from build123d import *

# Parameters (mm, degrees)
SKETCH1_R           = 1.5
SKETCH1_R_2         = 2.5
BOSS_EXTRUDE1_DEPTH = 3
CUT_EXTRUDE1_DEPTH  = 3
FILLET1_R           = 3
CHAMFER4_SIZE       = 15
CHAMFER5_DEPTH      = 3
SKETCH8_R           = 2
CUT_EXTRUDE4_DEPTH  = 10
SKETCH10_W          = 65
SKETCH10_H          = 15
BOSS_EXTRUDE2_DEPTH = 3
SKETCH9_W           = 6
SKETCH9_H           = 5
CUT_EXTRUDE5_DEPTH  = 10
FILLET2_R           = 3
SKETCH11_W          = 40
SKETCH11_H          = 3
CUT_EXTRUDE6_DEPTH  = 10


with BuildPart() as part:
    # Sketch1 → Boss-Extrude1 (new body)
    with BuildSketch(Plane.XY):
        with BuildLine():
            Line((40.5, -40), (44.5, -40))
            Line((44.5, -40), (47.5, -37))
            Line((47.5, -37), (47.5, 10))
            Line((47.5, 10), (47.5, 15))
            Line((47.5, 15), (52.5, 15))
            Line((52.5, 15), (70, 15))
            ThreePointArc((70, 15), (73.535533906, 16.464466094), (75, 20))
            Line((75, 20), (75, 60))
            ThreePointArc((75, 60), (73.535533906, 63.535533906), (70, 65))
            Line((70, 65), (-70, 65))
            ThreePointArc((-70, 65), (-73.535533906, 63.535533906), (-75, 60))
            Line((-75, 60), (-75, 20))
            ThreePointArc((-75, 20), (-73.535533906, 16.464466094), (-70, 15))
            Line((-70, 15), (-52.5, 15))
            Line((-52.5, 15), (-47.5, 15))
            Line((-47.5, 15), (-47.5, 10))
            Line((-47.5, 10), (-47.5, -37))
            Line((-47.5, -37), (-44.5, -40))
            Line((-44.5, -40), (-40.5, -40))
            Line((-40.5, -40), (-37.5, -37))
            Line((-37.5, -37), (-37.5, 10))
            ThreePointArc((-37.5, 10), (-36.035533906, 13.535533906), (-32.5, 15))
            Line((-32.5, 15), (32.5, 15))
            ThreePointArc((32.5, 15), (36.035533906, 13.535533906), (37.5, 10))
            Line((37.5, 10), (37.5, -37))
            Line((37.5, -37), (40.5, -40))
        make_face()
        with Locations((-42.5, -20)):
            Circle(SKETCH1_R, mode=Mode.SUBTRACT)
        with Locations((-42.5, -35)):
            Circle(SKETCH1_R, mode=Mode.SUBTRACT)
        with Locations((42.5, -20)):
            Circle(SKETCH1_R, mode=Mode.SUBTRACT)
        with Locations((42.5, -35)):
            Circle(SKETCH1_R, mode=Mode.SUBTRACT)
        with Locations((60, 40)):
            Circle(SKETCH1_R_2, mode=Mode.SUBTRACT)
        with Locations((15, 60)):
            Circle(SKETCH1_R, mode=Mode.SUBTRACT)
        with Locations(Location((-15, 60, 0), (0, 0, 180))):
            Circle(SKETCH1_R, mode=Mode.SUBTRACT)
        with Locations(Location((-60, 40, 0), (0, 0, 180))):
            Circle(SKETCH1_R_2, mode=Mode.SUBTRACT)
    extrude(amount=BOSS_EXTRUDE1_DEPTH)

    # Sketch3 → Cut-Extrude1 (cut)
    with BuildSketch(Plane.XY.offset(3)):
        Polygon((65, 50), (65, 30), (47.5, 30), (47.5, 15), (75, 15), (75, 23.034767996), (75, 32.364095159), (75, 65), (47.5, 65), (47.5, 50), align=None)
        Polygon((-47.5, 65), (-75, 65), (-75, 32.364095159), (-75, 23.034767996), (-75, 15), (-47.5, 15), (-47.5, 30), (-65, 30), (-65, 50), (-47.5, 50), align=None)
    extrude(amount=-CUT_EXTRUDE1_DEPTH, mode=Mode.SUBTRACT)

    # Fillet1
    fillet1_edges = [part.edges().sort_by_distance(p)[0] for p in [
        (65, 50, 1.5),
        (65, 30, 1.5),
        (-65, 50, 1.5),
        (-65, 30, 1.5),
    ]]
    fillet(fillet1_edges, radius=FILLET1_R)

    # Chamfer4
    chamfer4_edges = [part.edges().sort_by_distance(p)[0] for p in [
        (47.5, 65, 1.5),
        (-47.5, 65, 1.5),
    ]]
    chamfer(chamfer4_edges, length=CHAMFER4_SIZE - 0.0001)  # a hair under: the kernel refuses the full size

    # Chamfer5: read off the stored shape, not the designer's step
    # Chamfer5 outline → Chamfer5 (add)
    with BuildSketch(Plane.XY):
        with BuildLine():
            Line((47.5, 15.006945785), (62.083333333, 30.001157631))
            ThreePointArc((62.083333333, 30.001157631), (62.041670687, 30.000289422), (62, 30))
            Line((62, 30), (47.5, 30))
            Line((47.5, 30), (47.5, 15.006945785))
        make_face()
        with BuildLine():
            Line((-62.083333333, 30.001157631), (-47.5, 15.006945785))
            Line((-47.5, 15.006945785), (-47.5, 30))
            Line((-47.5, 30), (-62, 30))
            ThreePointArc((-62, 30), (-62.041670687, 30.000289422), (-62.083333333, 30.001157631))
        make_face()
    extrude(amount=CHAMFER5_DEPTH)

    # Sketch8 → Cut-Extrude4 (cut)
    with BuildSketch(Plane.XY.offset(3)):
        with Locations((-17.5, 43.444515249)):
            Circle(SKETCH8_R)
        with Locations((17.5, 43.444515249)):
            Circle(SKETCH8_R)
    extrude(amount=-CUT_EXTRUDE4_DEPTH, mode=Mode.SUBTRACT)

    # Sketch10 → Boss-Extrude2 (add)
    with BuildSketch(Plane.XY.offset(3)):
        with Locations((0, 72.5)):
            Rectangle(SKETCH10_W, SKETCH10_H)
    extrude(amount=-BOSS_EXTRUDE2_DEPTH)

    # Sketch9 → Cut-Extrude5 (cut)
    with BuildSketch(Plane.XY.offset(3)):
        with Locations((-25.5, 74.5)):
            Rectangle(SKETCH9_W, SKETCH9_H)
        with Locations((25.5, 74.5)):
            Rectangle(SKETCH9_W, SKETCH9_H)
    extrude(amount=-CUT_EXTRUDE5_DEPTH, mode=Mode.SUBTRACT)

    # Fillet2
    fillet2_edges = [part.edges().sort_by_distance(p)[0] for p in [
        (-32.5, 80, 1.5),
        (32.5, 80, 1.5),
    ]]
    fillet(fillet2_edges, radius=FILLET2_R)

    # Sketch11 → Cut-Extrude6 (cut)
    with BuildSketch(Plane.XY.offset(3)):
        with Locations((0, 20.5)):
            Rectangle(SKETCH11_W, SKETCH11_H)
    extrude(amount=-CUT_EXTRUDE6_DEPTH, mode=Mode.SUBTRACT)


solid = part.part
Model file for the job. Use its own axes, mm. A direction names the side the tool comes from. Give positions to 0.01 mm unless a question says otherwise; leave off trailing zeros. Loops run counter-clockwise (first coordinate to the right, second up) from the corner with the lowest first, then second, coordinate; pieces in that order, holes last.
1) Wall check: line 1 (Y direction, x = -15, z = 0.9); line 2 (X direction, y = 73, z = 0.55); line 3 (Y direction, x = -11, z = 1.25). Give the ranges that are in metal, low to high.
2) Tool access for faces 4 (the flat face through (65, 40, 2)), 5 (the flat face through (0, 15, 1)), 6 (the cylindrical face through (64.1, 49.14, 1.48)), 7 (the flat face through (-32.5, 71, 2)), 8 (the flat face through (-26, 72, 2)): list every direction of +Z, -Z, +X, -X, +Y, -Y with a clear straight run to the whole face (end or side of a thin tool).
3) Saw through at A-A (y = -35). Write the cut outline in (x, z).
4) Pull direction Y, two halves, no side cores. Call faces 1 (the cylindrical face through (41.39, -18.99, 1.48)), 2 (the flat face through (39.9, 57.6, 1.5)), 3 (the flat face through (-1, 34, 0)): +Y half, -Y half, draft (parallel to the pull), parting line (faces both ways), or undercut.
5) Saw through at D-D (x = -42.5). Write the cut outline in (y, z), plus the area to 3 significant figures.
6) Saw through at C-C (x = 60). Write the cut outline in (y, z), plus the area to 3 significant figures.
7) Flat gauge pins, fed straight in: pin 1 Ø0.9 at (x, z) = (-53.5, 1.5) entering from +Y; pin 2 Ø1.5 at (y, z) = (69, 1.5) entering from -X; pin 3 Ø8 at (x, y) = (60, 40) entering from -Z; pin 4 Ø0.9 at (y, z) = (68.5, 1.5) entering from +X. Where does each tip first touch, or does it go through?
8) Saw through at B-B (y = -14.5). Write the cut outline in (x, z), plus the area to 3 significant figures.
Answer block:
1. line 1: y = 15 to 19, 22 to 58.5, 61.5 to 80
1. line 2: x = -32.5 to -28.5, -22.5 to 22.5, 28.5 to 32.5
1. line 3: y = 15 to 19, 22 to 80
2. face 4: +Z, -Z, +X, +Y, -Y
2. face 5: +Z, -Z, -Y
2. face 6: +Z, -Z, +X, +Y
2. face 7: +Z, -Z, -X, +Y
2. face 8: +Z, -Z
3. outline: (-47.5, 0) - (-44, 0) - (-44, 3) - (-47.5, 3) - close; (-41, 0) - (-37.5, 0) - (-37.5, 3) - (-41, 3) - close; (37.5, 0) - (41, 0) - (41, 3) - (37.5, 3) - close; (44, 0) - (47.5, 0) - (47.5, 3) - (44, 3) - close
4. face 1: undercut
4. face 2: +Y half
4. face 3: draft
5. outline: (-40, 0) - (-36.5, 0) - (-36.5, 3) - (-40, 3) - close; (-33.5, 0) - (-21.5, 0) - (-21.5, 3) - (-33.5, 3) - close; (-18.5, 0) - (55, 0) - (55, 3) - (-18.5, 3) - close
5. area: 267 mm2
6. outline: (27.86, 0) - (37.5, 0) - (37.5, 3) - (27.86, 3) - close; (42.5, 0) - (50, 0) - (50, 3) - (42.5, 3) - close
6. area: 51.4 mm2
7. pin 1: stops at y = 50
7. pin 2: stops at x = -32.5
7. pin 3: stops at z = 0
7. pin 4: stops at x = 32.5
8. outline: (-47.5, 0) - (-37.5, 0) - (-37.5, 3) - (-47.5, 3) - close; (37.5, 0) - (47.5, 0) - (47.5, 3) - (37.5, 3) - close
8. area: 60.0 mm2
